Source: three-view drawing plus pictorial views. Frame: mm from the lowest corner of the part. Coordinates: 2 decimals unless noted, no trailing zeros. Loops run counter-clockwise (first coordinate to the right, second up) from the corner with the lowest first, then second, coordinate; pieces in that order, holes last. Notation, with made-up numbers: (-36.75, 78) -> (5.25, 78) arc R14 ccw to (5.25, 91) -> close; hole circle Ø7 at (29.25, 56.25). An arc over 180 degrees is marked (long way). Answer as a JSON object with one key per item and string values. Group by question number.
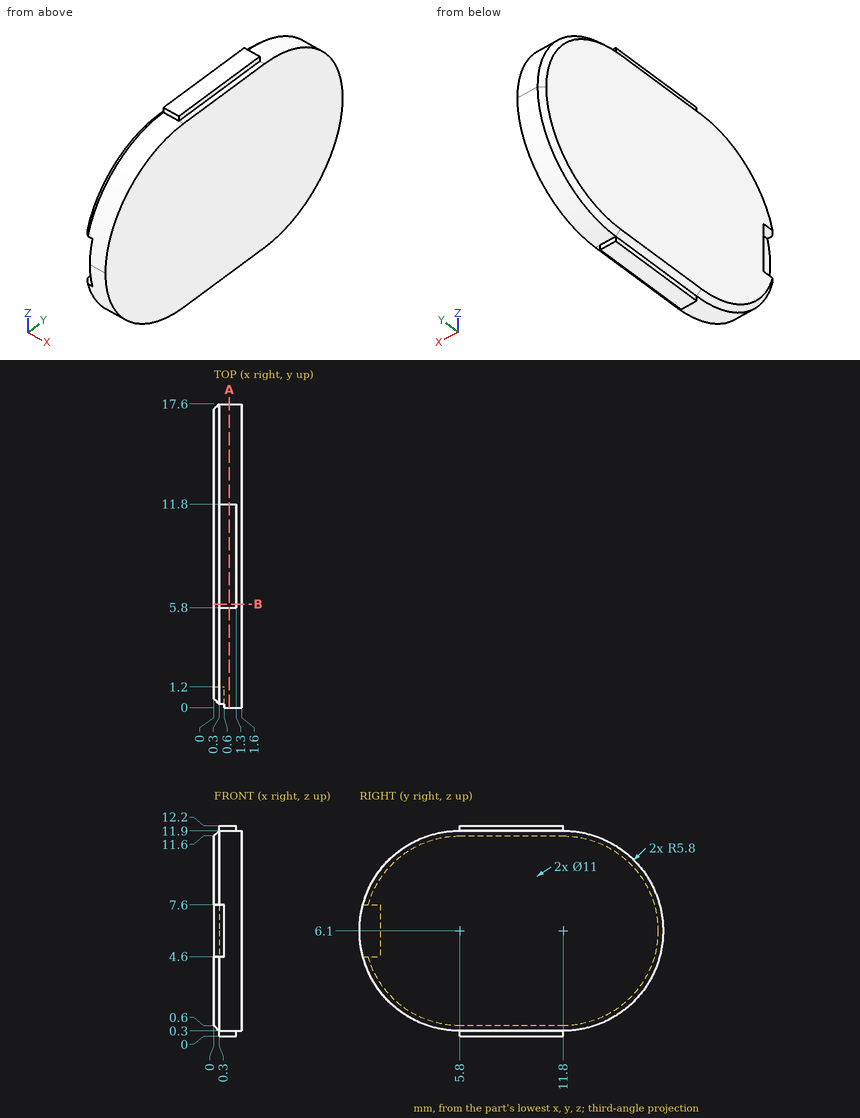
1. Pin query (flat end, axial travel): pin 1 Ø0.7 at (x, y) = (0.5, 1) entering from +Z; pin 2 Ø0.7 at (x, z) = (0, 6) entering from -Y; pin 3 Ø0.7 at (x, y) = (0, 1) entering from -Z. Return the tip coordinate at first contact, or that it passes through.
2. Section query B-B on y = 6. Return loops of the section in (x, z).
3. Ray query, L1, parallel to Z at x = 1.45, y = 11.75; L2, parallel to Y at x = 1, z = 5.25; L3, parallel to Y at x = 1, z = 4.25. Return the intervals inside material, ascending.
4. Section query A-A on x = 0.9. Return loops of the section in (y, z), then the cut area to 3 significant figures.
Solved:
{
 "1": {"pin 1": "z = 9.82", "pin 2": "y = 1.2", "pin 3": "z = 2.59"},
 "2": {"outline": "(0, 0.6) -> (0.3, 0.3) -> (0.3, 0) -> (1.3, 0) -> (1.3, 0.3) -> (1.6, 0.3) -> (1.6, 11.9) -> (1.3, 11.9) -> (1.3, 12.2) -> (0.3, 12.2) -> (0.3, 11.9) -> (0, 11.6) -> close"},
 "3": {"L1": "0.3 to 11.9", "L2": "0.06 to 17.54", "L3": "0.3 to 17.3"},
 "4": {"outline": "(5.8, 0) -> (11.8, 0) -> (11.8, 0.3) arc R5.8 ccw to (11.8, 11.9) -> (11.8, 12.2) -> (5.8, 12.2) -> (5.8, 11.9) arc R5.8 ccw to (5.8, 0.3) -> close", "area": "179 mm^2"}
}
